CAD build for the part. Positions are in the model's coordinates, mm. A direction names the side the tool comes from. Round coordinates to 2 decimals unless told otherwise and drop trailing zeros. Order: outer loops, then holes, each group sorted by start corner. A loop starts at its lowest first (then second) coordinate and runs counter-clockwise, first axis right, second up. Notation, with made-up numbers: (-3.75, -8.75) - (28.25, -8.75) arc R18 cw to (28.25, 3.25) - close; hole circle Ø10 at (66, -13). An arc over 180 degrees is marked (long way). Write item = value, one per line.
Autodesk Inventor part; units mm, degrees
ref_plane "YZ Plane" through (0, 0, 0) normal (1, 0, 0) x (0, 1, 0)
ref_plane "XZ Plane" through (0, 0, 0) normal (0, 1, 0) x (-1, 0, 0)
ref_plane "XY Plane" through (0, 0, 0) normal (0, 0, 1) x (1, 0, 0)
sketch "スケッチ1" plane through (0, 0, 0) normal (1, 0, 0) x (0, 1, 0)
  line L0 (37.123, 0) -> (-35.25, 0)
  line L1 (-35.25, 0) -> (-35.25, -80)
  line L2 (-35.25, -80) -> (37.123, -80)
  line L3 (37.123, -80) -> (37.123, 0)
  line L4 (-35.25, 0) -> (-35.25, -17.883)
  line L5 (37.123, 0) -> (37.123, -13.85)
  line L6 (37.123, -13.85) -> (22.5, -80)
  line L7 (-35.25, -17.883) -> (-24.5, -80)
  circle A0 centre (0, 0) radius 9.85
  line L8 (0, 0) -> (0, -80)
  line L9 (14.5, -80) -> (0, -80)
  line L10 (0, -80) -> (0, -75)
  line L11 (0, -75) -> (14.5, -75)
  line L12 (14.5, -75) -> (14.5, -80)
  line L13 (0, -75) -> (-14.5, -75)
  line L14 (-14.5, -75) -> (-14.5, -80)
  circle A1 centre (0, -20.151) radius 4
  circle A2 centre (0, -64.253) radius 4
  line L15 (4, -20.151) -> (4, -64.253)
  line L16 (-4, -64.253) -> (-4, -20.151)
  line L17 (11.25, 0) -> (-35.25, 0)
  line L18 (-35.25, 0) -> (-35.25, -14.25)
  line L19 (-35.25, -14.25) -> (11.25, -14.25)
  line L20 (11.25, -14.25) -> (11.25, 0)
  circle A3 centre (17, -22.151) radius 3.1
  line L21 (17, -22.151) -> (17, -58.151)
  circle A4 centre (17, -58.151) radius 3.1
  line L22 (20.1, -22.151) -> (20.1, -58.151)
  line L23 (13.9, -58.151) -> (13.9, -22.151)
  circle A5 centre (-17, -22.151) radius 3.1
  line L24 (-17, -22.151) -> (-17, -62.151)
  circle A6 centre (-17, -62.151) radius 3.1
  line L25 (-13.9, -22.151) -> (-13.9, -62.151)
  line L26 (-20.1, -22.151) -> (-20.1, -62.151)
  line L27 (-35.25, 0) -> (-35.25, 80)
  line L28 (-35.25, 80) -> (37.123, 80)
  line L29 (37.123, 80) -> (37.123, 0)
  line L30 (-35.25, 0) -> (-35.25, 17.883)
  line L31 (37.123, 0) -> (37.123, 13.85)
  line L32 (37.123, 13.85) -> (22.5, 80)
  line L33 (-35.25, 17.883) -> (-24.5, 80)
  circle A7 centre (0, 20.151) radius 4
  circle A8 centre (0, 64.253) radius 4
  line L34 (4, 20.151) -> (4, 64.253)
  line L35 (-4, 64.253) -> (-4, 20.151)
  circle A9 centre (17, 22.151) radius 3.1
  line L36 (17, 22.151) -> (17, 58.151)
  circle A10 centre (17, 58.151) radius 3.1
  line L37 (20.1, 22.151) -> (20.1, 58.151)
  line L38 (13.9, 58.151) -> (13.9, 22.151)
  circle A11 centre (-17, 22.151) radius 3.1
  circle A12 centre (-17, 62.151) radius 3.1
  line L39 (-13.9, 22.151) -> (-13.9, 62.151)
  line L40 (-20.1, 22.151) -> (-20.1, 62.151)
  dimension "d0" = 72.373
  dimension "d1" = 37.123
  dimension "d2" = 80
  dimension "d3" = 17.883
  dimension "d4" = 13.85
  dimension "d7" = 19.7
  dimension "d8" = 14.5
  dimension "d9" = 5
  dimension "d10" = 8
  dimension "d11" = 10
  dimension "d12" = 8
  dimension "d13" = 20.151
  dimension "d14" = 8
  dimension "d15" = 15.747
  dimension "d16" = 11.25
  dimension "d17" = 14.25
  dimension "d18" = 6.2
  dimension "d19" = 17
  dimension "d20" = 22.151
  dimension "d21" = 36
  dimension "d22" = 6.2
  dimension "d23" = 6.2
  dimension "d24" = 22.151
  dimension "d25" = 17
  dimension "d26" = 40
  dimension "d27" = 6.2
extrude "押し出し1" add sketch "スケッチ1" along normal blind 1.5 contours L3 L6 L2 L12 L11 L8 A2 L15 A1 L19 L20 L0 | L0 A0 L27 L33 L28 L32 L29 | L20 L19 L8 A0 L0 | A0 L8 L19 L1 L0 | L8 A1 L16 A2 L13 L14 L2 L7 L1 L19 | L2 L8 L11 L12 | L2 L14 L13 L8
sketch "スケッチ2" plane through (1.5, 0, 0) normal (1, 0, 0) x (0, 0, -1)
  line L0 (-17.883, -35.25) -> (17.883, -35.25)
  line L1 (0, 11.25) -> (14.25, 11.25)
  line L2 (14.25, 11.25) -> (14.25, -35.25)
  line L3 (14.25, -35.25) -> (0, -35.25)
  line L4 (0, -35.25) -> (0, 11.25)
  circle A0 centre (0, 0) radius 9.85
  point P0 (11, 8)
  point P1 (11, -32)
  point P2 (-11, 8)
  point P3 (-11, -32)
  dimension "d30" = 14.25
  dimension "d31" = 11.25
  dimension "d32" = 3.25
  dimension "d33" = 3.25
  dimension "d34" = 3.25
  dimension "d35" = 3.25
hole "穴1" at (1.5, 8, -11) at (1.5, -32, -11) at (1.5, 8, 11) at (1.5, -32, 11) direction (-1, 0, 0) diameter 2.5 end through all
sketch "スケッチ3" plane through (1.5, 0, 0) normal (1, 0, 0) x (0, 0, -1)
  line L0 (0, 0) -> (80, 0)
  line L1 (80, -24.5) -> (80, 22.5)
  line L2 (13.85, 37.123) -> (-13.85, 37.123)
  line L3 (0, 37.123) -> (0, -35.25)
  line L4 (-17.883, -35.25) -> (17.883, -35.25)
  point P0 (75, 14.5)
  point P1 (75, -14.5)
  point P2 (-75, 14.5)
  point P3 (-75, -14.5)
  dimension "d43" = 5
  dimension "d44" = 14.5
hole "穴2" at (1.5, 14.5, -75) at (1.5, -14.5, -75) at (1.5, 14.5, 75) at (1.5, -14.5, 75) direction (-1, 0, 0) diameter 2.1 end through all
fillet "フィレット1" radius 5 4 edges at (0.75, 22.5, -80) (0.75, -24.5, -80) (0.75, 22.5, 80) (0.75, -24.5, 80)
sketch "スケッチ4" plane through (0, 0, 0) normal (-1, 0, 0) x (0, 0, 1)
  circle A0 centre (0, 0) radius 27.5
  arc A1 (-22.151, 13.9) -> (-22.151, 20.1) centre (-22.151, 17) ccw
  circle A2 centre (-22.151, 17) radius 3.1
  arc A3 (22.151, -13.9) -> (22.151, -20.1) centre (22.151, -17) ccw
  circle A4 centre (22.151, -17) radius 3.1
  arc A5 (-22.151, -20.1) -> (-22.151, -13.9) centre (-22.151, -17) ccw
  circle A6 centre (-22.151, -17) radius 3.1
  arc A7 (22.151, 20.1) -> (22.151, 13.9) centre (22.151, 17) ccw
  circle A8 centre (22.151, 17) radius 3.1
  circle A9 centre (0, 0) radius 24.8225
  circle A10 centre (0, 0) radius 31.0225
  line L0 (0, 0) -> (8.0292, 29.9654)
  line L1 (0, 0) -> (0, 31.0225)
  line L2 (0, 0) -> (-8.0292, -29.9654)
  circle A11 centre (7.2269, 26.9711) radius 3.1
  circle A12 centre (-7.2269, -26.9711) radius 3.1
  line L3 (0, 0) -> (13.1107, -28.1159)
  circle A13 centre (11.8006, -25.3064) radius 3.1
  line L4 (0, 0) -> (-13.1107, 28.1159)
  circle A14 centre (-11.8006, 25.3064) radius 3.1
  point P0 (19.6918, -15.1126)
  point P1 (-19.6918, -15.1126)
  point P2 (-24.6102, -18.8874)
  point P3 (24.6102, -18.8874)
  point P4 (24.6102, 18.8874)
  point P5 (-24.6102, 18.8874)
  point P6 (-22.151, 20.1)
  point P7 (-19.6918, 15.1126)
  point P8 (19.6918, 15.1126)
  point P9 (22.151, 20.1)
  point P10 (-8.0292, -29.9654)
  point P11 (-6.4245, -23.9767)
  point P12 (8.0292, 29.9654)
  point P13 (6.4245, 23.9767)
  point P14 (10.4904, -22.4968)
  point P15 (-10.4904, 22.4968)
  dimension "d53" = 55
  dimension "d56" = 15
  dimension "d57" = 25
extrude "押し出し2" cut sketch "スケッチ4" against normal blind 10 contours A4 A3 A0 | A0 A3 A4 | A3 A4 A10 A13 A0 | A0 A13 A9 A3 | A13 L3 A0 | A0 L3 A13 | L3 A13 A0 | A0 A13 L3 | A14 A0 L4 | A9 A1 A0 A14 | L4 A0 A14 | A14 A0 A1 A2 A10 | A14 A0 L4 | L4 A0 A14 | A1 A2 A0 | A2 A1 A0
equation "\"BendRadius\" = Thickness"
equation "\"BendReliefWidth\" = Thickness"
equation "\"BendReliefDepth\" = 0.5 * Thickness"
equation "\"CornerReliefSize\" = 4 * Thickness"
equation "\"MinimumRemnant\" = 2 * Thickness"
equation "\"TransitionRadius\" = BendRadius"
equation "\"JacobiRadiusSize\" = BendRadius"
equation "\"GapSize\" = Thickness"
properties part number "joint_adaptor_plate" material "アルミニウム 6061"
(1) Pull direction Z, two halves, no side cores. Call faces 1 (the cylindrical face through (0.74, -0.09, 68.25)), 2 (the cylindrical face through (0.74, 24.73, -18.73)), 3 (the cylindrical face through (0.76, -23.55, -78.79)), 4 (the cylindrical face through (0.76, -23.47, 78.86)): released by +Z, released by -Z, zero draft, split by the parting line, or undercut.
Solved:
face_1 = undercut
face_2 = undercut
face_3 = released by -Z
face_4 = released by +Z
(2) Band-saw the part on B-B on z = 28. List the corners of the cut face in (x, y), plus the area to 3 significant figures.
Solved:
outline = (0, -33.5) - (1.5, -33.5) - (1.5, -20.1) - (0, -20.1) - close; (0, -13.9) - (1.5, -13.9) - (1.5, -4) - (0, -4) - close; (0, 4) - (1.5, 4) - (1.5, 13.9) - (0, 13.9) - close; (0, 20.1) - (1.5, 20.1) - (1.5, 34) - (0, 34) - close
area = 70.6 mm²
(3) Probe line 1 along Z through (x, y) = (1.4, 15); line 2 along Y through (x, z) = (0.55, -75); line 3 along Z through (x, y) = (1.15, 14.5). List the from-to ranges inside material, lowest first.
Solved:
line_1 = -80 to -75.92, -74.08 to -60.52, -19.78 to 19.78, 60.52 to 74.08, 75.92 to 80
line_2 = -25.37 to -15.55, -13.45 to 13.45, 15.55 to 23.61
line_3 = -80 to -76.05, -73.95 to -59.98, -20.32 to 20.32, 59.98 to 73.95, 76.05 to 80
(4) Drop flat-ended pins along their axis: pin 1 (1.3 mm diameter, centred on y = 14.5, z = -75, fed in from +X); pin 2 (3 mm diameter, centred on y = -32, z = 11, fed in from +X); pin 3 (0.8 mm diameter, centred on x = 1, z = 48.5, fed in from -Y); pin 4 (0.8 mm diameter, centred on x = 0.5, z = 38, fed in from +Y). Give the stop position or say it passes through.
Solved:
pin_1 = through
pin_2 = 1.5
pin_3 = -30.02
pin_4 = 31.87
(5) Band-saw the part on C-C on y = 1. List the corners of the cut face in (x, z), plus the area to 3 significant figures.
Solved:
outline = (0, -80) - (1.5, -80) - (1.5, -68.13) - (0, -68.13) - close; (0, -16.28) - (1.5, -16.28) - (1.5, -9.8) - (0, -9.8) - close; (0, 9.8) - (1.5, 9.8) - (1.5, 16.28) - (0, 16.28) - close; (0, 68.13) - (1.5, 68.13) - (1.5, 80) - (0, 80) - close
area = 55.1 mm²
(6) Band-saw the part on A-A on z = 0. List the corners of the cut face in (x, y).
Solved:
outline = (0, -35.25) - (1.5, -35.25) - (1.5, -9.85) - (0, -9.85) - close; (0, 9.85) - (1.5, 9.85) - (1.5, 37.12) - (0, 37.12) - close
(7) Band-saw the part on D-D on y = 17. List the corners of the cut face in (x, z), plus the area to 3 significant figures.
Solved:
outline = (0, -80) - (1.5, -80) - (1.5, -61.25) - (0, -61.25) - close; (0, -18.09) - (1.5, -18.09) - (1.5, 19.05) - (0, 19.05) - close; (0, 61.25) - (1.5, 61.25) - (1.5, 80) - (0, 80) - close
area = 112 mm²
(8) Tool access for faces 5 (the cylindrical face through (0.76, 21.65, 78.87)), 6 (the cylindrical face through (0.74, 0.088, 16.152)): list every direction of +Z, -Z, +X, -X, +Y, -Y with a clear straight run to the whole face (end or side of a thin tool).
Solved:
face_5 = +Z, +X, -X, +Y
face_6 = +X, -X
